Read the model definition and answer for the solid it produces. Units are mm, in the model's axes. Face numbers are marked on the shaded views. A direction names the side the tool comes from. Give positions to 0.01 mm unless a question says otherwise; leave off trailing zeros. Order: outer loops, then holes, each group sorted by start corner. A loop starts at its lowest first (then second) coordinate and runs counter-clockwise, first axis right, second up. Notation, with made-up numbers: (82.25, 80.25) - (112.25, 80.25) arc R32 ccw to (112.25, 118.25) - close; hole circle Ø7 at (-19.75, -2). An arc over 180 degrees is marked (long way). Use a Markdown table: item, result. Add a question column.
1. A cutting plane is placed at A-A on z = 3.5. Determine the outline of the cut face in (x, y), and give its area (3 significant figures).
2. Consider L1, parallel to X at y = -14, z = 5.75; L2, parallel to Y at x = -26, z = 4; L3, parallel to Y at x = -4, z = 10.5. Determine where each line is inside the solid, lowest interval first.
3. A cutting plane is placed at B-B on y = -25. Determine the outline of the cut face in (x, z), and give its area (3 significant figures).
4. For a pull along X with two mould halves and no side action, classify the marked faces 1, 2 and 3 as released by +X, released by -X, zero draft, split by the parting line, or undercut.
5. Which of the six approach directions +Z, -Z, +X, -X, +Y, -Y give full straight-line access (tool end or side, diameter ignored) to the marked faces 4, 5 and 6?
6. Flat-ended cylindrical pins translate along their axes: P1, Ø2, axis at x = 31, z = 7, coming from the +Y side; P2, Ø5, axis at x = 10, y = 22.5, coming from the +Z side; P3, Ø2, axis at x = 25, z = 3, coming from the +Y side. Find the tip coordinate at first contact, or state that the pin passes through.
7. A cutting plane is placed at C-C on x = 4.5. Determine the outline of the cut face in (y, z).
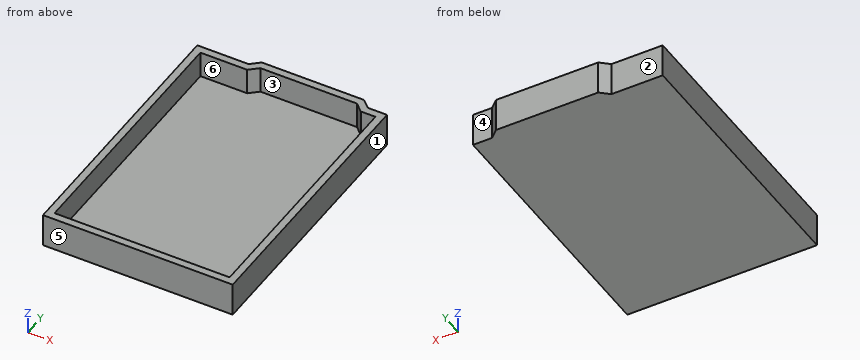
```python
from build123d import *

# Parameters (mm, degrees)
F1_DEPTH = 11.684
F2_T     = -2.54


with BuildPart() as f1:
    # F0 (on Top) → F1 (new body)
    with BuildSketch(Plane.XY):
        Polygon((-14.5989814773, 38.1090268493), (-32.4211120605, 38.1090268493), (-32.4211120605, -54.6039827168), (33.3690978587, -54.6039827168), (33.3690978587, 38.1090268493), (26.7332009971, 38.1090268493), align=None)
        Polygon((-11.5654272959, 40.7633893192), (-14.5989814773, 38.1090268493), (26.7332009971, 38.1090268493), (23.8892417401, 40.7633893192), align=None)
    extrude(amount=F1_DEPTH)

    # F2
    f2_openings = [f1.faces().sort_by_distance(p)[0] for p in [
        (0.566664, -7.464444, 11.684),
    ]]
    offset(amount=F2_T, openings=f2_openings, kind=Kind.INTERSECTION)


solid = f1.part
```
Output values:
| question | item | result |
|---|---|---|
| 1 | outline | (-32.42, -54.6) - (33.37, -54.6) - (33.37, 38.11) - (26.73, 38.11) - (23.89, 40.76) - (-11.57, 40.76) - (-14.6, 38.11) - (-32.42, 38.11) - close; hole (-29.88, -52.06) - (30.83, -52.06) - (30.83, 35.57) - (25.73, 35.57) - (22.89, 38.22) - (-10.61, 38.22) - (-13.64, 35.57) - (-29.88, 35.57) - close |
| 1 | area | 785 mm² |
| 2 | L1 | -32.42 to -29.88, 30.83 to 33.37 |
| 2 | L2 | -54.6 to -52.06, 35.57 to 38.11 |
| 2 | L3 | -54.6 to -52.06, 38.22 to 40.76 |
| 3 | outline | (-32.42, 0) - (33.37, 0) - (33.37, 11.68) - (30.83, 11.68) - (30.83, 2.54) - (-29.88, 2.54) - (-29.88, 11.68) - (-32.42, 11.68) - close |
| 3 | area | 214 mm² |
| 4 | face 1 | released by +X |
| 4 | face 2 | zero draft |
| 4 | face 3 | undercut |
| 5 | face 4 | +Z, -Z, +X, +Y |
| 5 | face 5 | +Z, -Z, +X, -X, -Y |
| 5 | face 6 | +Z |
| 6 | P1 | y = 38.11 |
| 6 | P2 | z = 2.54 |
| 6 | P3 | y = 40.66 |
| 7 | outline | (-54.6, 0) - (40.76, 0) - (40.76, 11.68) - (38.22, 11.68) - (38.22, 2.54) - (-52.06, 2.54) - (-52.06, 11.68) - (-54.6, 11.68) - close |
